from build123d import *

# Parameters (mm, degrees)
F0_W     = 95.1395854354
F0_H     = 35.537417978
F1_DEPTH = 50
F2_R     = 12.5
F3_T     = 2.5
F4_R     = 5
F5_R     = 4.25
F6_DEPTH = 25


# Not quite as in the source:
# - a shell that OpenCascade refuses in one call is made with other operations: the cavity is built on its own and cut out


with BuildPart() as f1:
    # F0 (on Front) → F1 (new body)
    with BuildSketch(Plane.XZ):
        with Locations((-14.7300325334, 39.2820779234)):
            Rectangle(F0_W, F0_H)
    extrude(amount=-F1_DEPTH)

    # F2
    f2_edges = [f1.edges().sort_by_distance(p)[0] for p in [
        (-14.730033, 0, 57.050787),
    ]]
    fillet(f2_edges, radius=F2_R)

    # F3: shell of thickness 2.5, made by hand


with BuildPart() as f3_core1:
    # F3_t2: copy of F1
    add(f1.part)

    # the walls: a layer under each face that stays
    f3_faces = [f3_core1.faces().sort_by_distance(p)[0] for p in [
        (-14.7300325334, 3.6611652352, 53.3896216773),
        (-14.7300325334, 50, 39.2820779234),
        (-14.7300325334, 0, 33.0320779234),
        (-14.7300325334, 25, 21.5133689344),
    ]]
    thicken(f3_faces, amount=-F3_T, mode=Mode.SUBTRACT)


with BuildPart() as f1_1:
    add(f1.part)

    # what is left inside the walls is the cavity
    f3_cavity = [f3_core1.part.solids().sort_by_distance(p)[0] for p in [
        (-14.730033, 32.5, 24.038369),
    ]]
    add(f3_cavity, mode=Mode.SUBTRACT)

    # F4
    f4_edges = [f1_1.edges().sort_by_distance(p)[0] for p in [
        (-14.730033, 47.5, 24.013369),
    ]]
    fillet(f4_edges, radius=F4_R)

    # F5 (on face) → F6 (cut)
    with BuildSketch(Plane(origin=(0, 0, 21.5133689344), x_dir=(1, 0, 0), z_dir=(0, 0, -1))):
        with Locations((17.8397601843, -15)):
            Circle(F5_R)
    extrude(amount=-F6_DEPTH, mode=Mode.SUBTRACT)


solid = f1_1.part
Source: CAD feature listing. Evaluate the final solid. Frame: model axes, mm. A direction names the side the tool comes from. Round coordinates to 2 decimals unless told otherwise and drop trailing zeros. Order: outer loops, then holes, each group sorted by start corner. A loop starts at its lowest first (then second) coordinate and runs counter-clockwise, first axis right, second up. Notation, with made-up numbers: (-21, 66.25) - (-14, 66.25) arc R15 cw to (-14, 84.25) - close; hole circle Ø6 at (-22, 43). An arc over 180 degrees is marked (long way). Use a Markdown table: item, result. Add a question column.
1. Section query B-B (z = 45.5). Return the cut outline in (x, y), then the cut area to 3 significant figures.
2. Mould query, pull axis X, two halves, no side actions, for faces 4 (the cylindrical face through (21.766, 16.628, 22.746)), 5 (the flat face through (-62.3, 25, 23)), 6 (the flat face through (-15, 50, 40)). Classes: +X half, -X half, draft (parallel to the pull), parting line (faces both ways), or undercut.
3. Set-up query: faces 1 (the cylindrical face through (-14.06, 46, 25.44)), 2 (the flat face through (32.84, 25, 23)), 3 (the cylindrical face through (-14.06, 5.51, 51.7)). Return all of +Z, -Z, +X, -X, +Y, -Y with unobstructed straight access to the full face (end or side cutting, diameter ignored); none if empty.
4. Section query D-D (y = 31). Return the cut outline in (x, z).
5. First-contact query: pin 1 (12 mm diameter, centred on x = 4, y = 30.5, fed in from +Z); pin 2 (5 mm diameter, centred on x = -24.5, y = 43.5, fed in from +Z); pin 3 (6 mm diameter, centred on y = 22.5, z = 29, fed in from +X). Flat tips, straight axial feed; report the tip coordinate or a pass-through.
6. Section query C-C (x = -36.5). Return the cut outline in (y, z), then the cut area to 3 significant figures.
7. Section query A-A (y = 15). Return the cut outline in (x, z), then the cut area to 3 significant figures.
8. Line query: probe 1 along X at (y, z) = (15, 22); probe 2 along Y at (x, z) = (-16.5, 41); probe 3 along Z at (x, y) = (-48.5, 33). Output: solid intervals per line, ascending.
Derived:
| question | item | result |
|---|---|---|
| 1 | outline | (-62.3, 0.04) - (32.84, 0.04) - (32.84, 2.55) - (-62.3, 2.55) - close; (-62.3, 47.5) - (32.84, 47.5) - (32.84, 50) - (-62.3, 50) - close |
| 1 | area | 477 mm2 |
| 2 | face 4 | undercut |
| 2 | face 5 | -X half |
| 2 | face 6 | draft |
| 3 | face 1 | +Z, +X, -X |
| 3 | face 2 | +Z, -Z, +X, +Y, -Y |
| 3 | face 3 | +X, -X |
| 4 | outline | (-62.3, 21.51) - (32.84, 21.51) - (32.84, 24.01) - (-62.3, 24.01) - close |
| 5 | pin 1 | z = 24.01 |
| 5 | pin 2 | z = 25.44 |
| 5 | pin 3 | through |
| 6 | outline | (0, 21.51) - (50, 21.51) - (50, 57.05) - (47.5, 57.05) - (47.5, 29.01) arc R5 cw to (42.5, 24.01) - (2.5, 24.01) - (2.5, 44.55) arc R10 cw to (12.5, 54.55) - (12.5, 57.05) arc R12.5 ccw to (0, 44.55) - close |
| 6 | area | 308 mm2 |
| 7 | outline | (-62.3, 21.51) - (13.59, 21.51) - (13.59, 24.01) - (-62.3, 24.01) - close; (22.09, 21.51) - (32.84, 21.51) - (32.84, 24.01) - (22.09, 24.01) - close |
| 7 | area | 217 mm2 |
| 8 | probe 1 | -62.3 to 13.59, 22.09 to 32.84 |
| 8 | probe 2 | 0 to 2.5, 47.5 to 50 |
| 8 | probe 3 | 21.51 to 24.01 |
